Part print with two shaded views. Sizes in mm from the minimum x, y, z corner. A direction names the side the tool comes from. Give positions to 0.01 mm unless a question says otherwise; leave off trailing zeros. Write each loop counter-clockwise with the first axis right and the second up, starting at its lowest first coordinate (ties: lowest second). Pieces come first, ordered by that corner, then holes. Notation, with made-up numbers: (38.25, -5) - (74.25, -5) arc R27 ccw to (74.25, 14) - close; hole circle Ø2 at (-23, 60.25). An arc over 180 degrees is marked (long way). Answer as a JSON object with one key per item and string values.
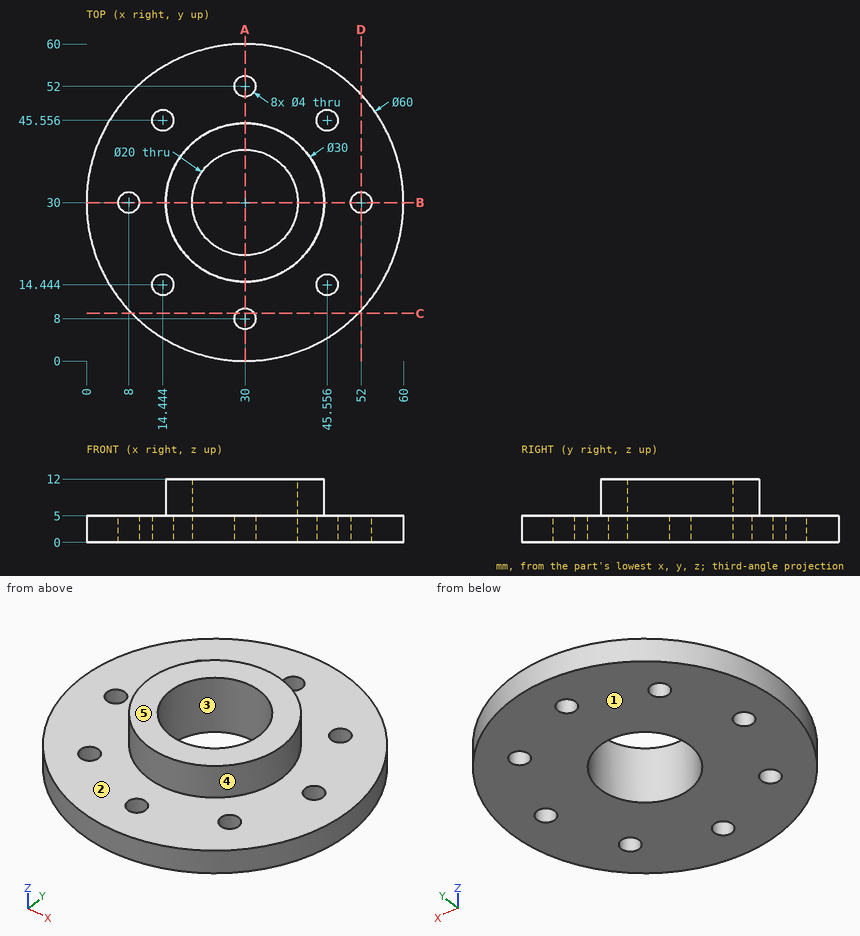
(1) Saw through at C-C, the plane y = 9. Give the cut face in (x, z), and give its area (3 significant figures).
Answer key:
{"outline": "(8.58, 0) - (28.27, 0) - (28.27, 5) - (8.58, 5) - close; (31.73, 0) - (51.42, 0) - (51.42, 5) - (31.73, 5) - close", "area": "197 mm²"}
(2) Pull direction Y, two halves, no side cores. Call the marked faces 3, 4 and 5: pulls with the +Y half, pulls with the -Y half, needs draft (parallel to the pull), parting line crosses it, or undercut.
Answer key:
{"face 3": "undercut", "face 4": "parting line crosses it", "face 5": "needs draft"}
(3) Flat gauge pins, fed straight in: P1, Ø3, axis at x = 14.44, y = 14.44, coming from the +Z side (3 decimals); P2, Ø2, axis at y = 9.5, z = 2.5, coming from the -X side; P3, Ø1, axis at x = 29.5, z = 9.5, coming from the +Y side; P4, Ø1.5, axis at x = 32.5, z = 6.5, coming from the -Y side. Where does each tip first touch, or does it go through?
Answer key:
{"P1": "passes through", "P2": "stops at x = 7.2", "P3": "stops at y = 45", "P4": "stops at y = 15.1"}
(4) Saw through at A-A, the plane x = 30. Give the cut face in (y, z).
Answer key:
{"outline": "(0, 0) - (6, 0) - (6, 5) - (0, 5) - close; (10, 0) - (20, 0) - (20, 12) - (15, 12) - (15, 5) - (10, 5) - close; (40, 0) - (50, 0) - (50, 5) - (45, 5) - (45, 12) - (40, 12) - close; (54, 0) - (60, 0) - (60, 5) - (54, 5) - close"}
(5) Saw through at D-D, the plane x = 52. Give the cut face in (y, z).
Answer key:
{"outline": "(9.6, 0) - (28, 0) - (28, 5) - (9.6, 5) - close; (32, 0) - (50.4, 0) - (50.4, 5) - (32, 5) - close"}
(6) Probe L1, parallel to Y at x = 14.5, z = 1.75 (1 decimal); L2, parallel to Y at x = 13, z = 3.5; L3, parallel to X at y = 30.5, z = 5.75. List the from-to ranges inside material, lowest first. Write a range as [from, to].
Answer key:
{"L1": "y = [4.3, 12.4], [16.4, 43.6], [47.6, 55.7]", "L2": "y = [5.28, 13.06], [15.83, 44.17], [46.94, 54.72]", "L3": "x = [15.01, 20.01], [39.99, 44.99]"}
(7) 3-axis set-ups, long thin cutter, end or side, ignore diameter. For the marked faces 1 and 2: which of +Z, -Z, +X, -X, +Y, -Y reach the whole face in a straight line?
Answer key:
{"face 1": "-Z, +X, -X, +Y, -Y", "face 2": "+Z"}
